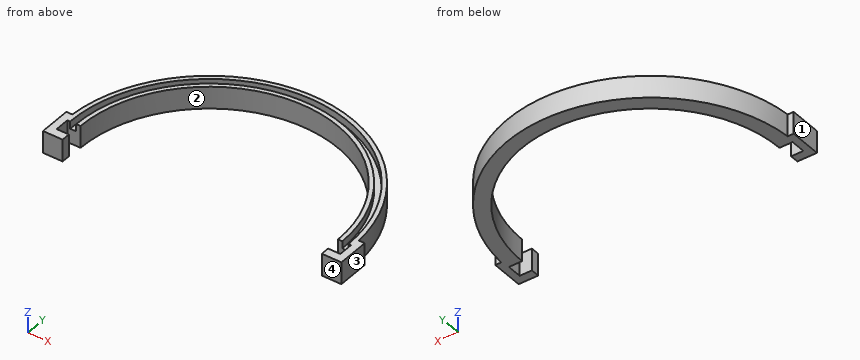
Solid Edge part; units mm, degrees
sketch "Sketch1" plane through (0, 0, 0) normal (0, -1, 0) x (1, 0, 0)
  line L0 (-117, 0) -> (-117, 18)
  line L1 (-117, 18) -> (-113.5, 18)
  line L2 (-113.5, 18) -> (-113.5, 12)
  line L3 (-113.5, 12) -> (-108.5, 12)
  line L4 (-108.5, 12) -> (-108.5, 18)
  line L5 (-108.5, 18) -> (-105, 18)
  line L6 (-105, 18) -> (-105, 0)
  line L7 (-105, 0) -> (-117, 0)
  dimension "D1" = 105
  dimension "D2" = 117
  dimension "D3" = 105
  dimension "D4" = 108.5
  dimension "D5" = 113.5
  dimension "D6" = 117
revolve "RevolvedProtrusion1" add sketch "Sketch1" angle 180 about axis through (0, 0, 54) along (0, 0, -1)
sketch "Sketch2" plane through (0, 58.5, 18) normal (0, 0, 1) x (1, 0, 0)
  line L0 (116.7904, -58.5) -> (116.7904, -51.5)
  line L1 (116.7904, -51.5) -> (121.6705, -51.5)
  line L2 (121.6705, -51.5) -> (121.6705, -77.5)
  line L3 (121.6705, -77.5) -> (105.6705, -77.5)
  line L4 (105.6705, -77.5) -> (105.6705, -70.5)
  line L5 (105.6705, -70.5) -> (115.6705, -70.5)
  line L6 (115.6705, -70.5) -> (115.6705, -58.5)
  line L7 (116.7904, -58.5) -> (115.6705, -58.5)
  dimension "D1" = 121.6705
  dimension "D2" = 115.6705
  dimension "D3" = 121.6705
extrude "ExtrudedProtrusion_3" add sketch "Sketch2" against normal blind 18
mirror "Mirror1" about plane through (0, 0, 0) normal (1, 0, 0) of "ExtrudedProtrusion_3"
properties material "ABS Plastic, high impact"
Input: part model. Units: mm. Frame: model coordinates. Face numbers are marked on the shaded views. Give positions to 0.01 mm unless a question says otherwise; leave off trailing zeros. Order: outer loops, then holes, each group sorted by start corner. A loop starts at its lowest first (then second) coordinate and runs counter-clockwise, first axis right, second up. Notation, with made-up numbers: M 68,49.25 L 79,49.25 A12 ccw 79,69.25 Z; hole C -8.5,74 d5. An arc over 180 degrees is marked long. Return JSON: item names as keys, results as strings.
Item 1: Cut plane C-C (y = 37). Return loops of the section in (x, z).
Solutions:
{"outline": "M -111,0 L -98.26,0 L -98.26,18 L -102,18 L -102,12 L -107.3,12 L -107.3,18 L -111,18 Z; M 98.26,0 L 111,0 L 111,18 L 107.3,18 L 107.3,12 L 102,12 L 102,18 L 98.26,18 Z"}
Item 2: Ray query, probe 1 along X at (y, z) = (-7.5, 6.25); probe 2 along X at (y, z) = (47, 17); probe 3 along X at (y, z) = (97.5, 14). Return the intervals inside material, ascending.
Solutions:
{"probe 1": "-121.67 to -115.67, 115.67 to 121.67", "probe 2": "-107.14 to -103.31, -97.79 to -93.89, 93.89 to 97.79, 103.31 to 107.14", "probe 3": "-64.67 to -58.1, -47.6 to -38.97, 38.97 to 47.6, 58.1 to 64.67"}
Item 3: Pull-direction query (X, two-part tool) for the marked faces 1, 2, 3 and 4; classes: +X half, -X half, draft (parallel to the pull), parting line (faces both ways), or undercut.
Solutions:
{"face 1": "-X half", "face 2": "undercut", "face 3": "+X half", "face 4": "draft"}
Item 4: First-contact query: P1, Ø1.5, axis at y = 76.5, z = 10, coming from the -X side; P2, Ø10, axis at y = 66.5, z = 14.5, coming from the +X side; P3, Ø1, axis at y = 21.5, z = 15.5, coming from the +X side. Flat tips, straight axial feed; report the tip coordinate or a pass-through.
Solutions:
{"P1": "x = -89.17", "P2": "x = 99.53", "P3": "x = 115.1"}
Item 5: Cut plane A-A (x = 0). Return loops of the section in (y, z).
Solutions:
{"outline": "M 105,0 L 117,0 L 117,18 L 113.5,18 L 113.5,12 L 108.5,12 L 108.5,18 L 105,18 Z"}
Item 6: Cut plane D-D (x = -32). Return loops of the section in (y, z) (3 decimals), then the cut area to 3 significant figures.
Solutions:
{"outline": "M 100.005,0 L 112.539,0 L 112.539,18 L 108.896,18 L 108.896,12 L 103.674,12 L 103.674,18 L 100.005,18 Z", "area": "194 mm^2"}
Item 7: Cut plane B-B (z = 3.5). Return loops of the section in (x, y), then the cut area to 3 significant figures.
Solutions:
{"outline": "M -121.67,-19 L -105.67,-19 L -105.67,-12 L -115.67,-12 L -115.67,0 L -105,0 A105 cw 105,0 L 115.67,0 L 115.67,-12 L 105.67,-12 L 105.67,-19 L 121.67,-19 L 121.67,7 L 116.79,7 A117 ccw -116.79,7 L -121.67,7 Z", "area": "4,620 mm^2"}
